Input: part model. Units: mm. Frame: model coordinates. A direction names the side the tool comes from. Round coordinates to 2 decimals unless told otherwise and drop trailing zeros. Loops run counter-clockwise (first coordinate to the right, second up) from the corner with the lowest first, then second, coordinate; pieces in that order, holes last. Notation, with made-up numbers: M -20.5,17 L 30.5,17 A23 cw 30.5,36 Z; hole C -37.5,-4 d2. An arc over 180 degrees is marked long. Use one line per item in the form item = value. Start each with the question number.
Q1. First-contact query: P1, Ø3, axis at x = -5, z = -6, coming from the +Y side; P2, Ø6, axis at y = 23.5, z = -13, coming from the -X side; P3, Ø4.5, axis at x = -4.5, z = -8.5, coming from the +Y side. Flat tips, straight axial feed; report the tip coordinate or a pass-through.
Q2. Section query A-A, the plane x = 0. Output: boundary loops of the cut face in (y, z), and give its area (3 significant figures).
Q3. Access query for faces 1 (the cylindrical face through (9.756, 13.804, -7.516)), 2 (the flat face through (0, 28, -11)). Directions: +Z, -Z, +X, -X, +Y, -Y. A direction counts if a zero-diameter tool reaches every point of the face in a straight line with its end or side. Return the directions, or none.
Q4. Section query D-D, the plane x = 4. Output: boundary loops of the cut face in (y, z), and give its area (3 significant figures).
Q5. Section query C-C, the plane y = 34. Output: boundary loops of the cut face in (x, z), and give its area (3 significant figures).
Q6. Section query B-B, the plane z = -7. Output: boundary loops of the cut face in (x, y).
Q7. Ray query, line 1 along Y through (x, z) = (6, -3.25); line 2 along X through (y, z) = (9.5, -7.5); line 3 along Y through (x, z) = (1, -5.5). Return the intervals inside material, ascending.
Autodesk Inventor part; units mm, degrees
ref_plane "YZ Plane" through (0, 0, 0) normal (1, 0, 0) x (0, 1, 0)
ref_plane "XZ Plane" through (0, 0, 0) normal (0, 1, 0) x (-1, 0, 0)
ref_plane "XY Plane" through (0, 0, 0) normal (0, 0, 1) x (1, 0, 0)
sketch "Sketch1" plane through (0, 0, 0) normal (0, 1, 0) x (-1, 0, 0)
  line L0 (0, 0) -> (-6.5, 0)
  line L1 (0, 0) -> (6.5, 0)
  line L2 (6.5, 0) -> (6.5, -15) construction
  line L3 (6.5, -15) -> (-7, -15)
  line L4 (-6.5, 0) -> (-9.5, 0) construction
  line L5 (6.5, 0) -> (9.5, 0) construction
  arc A0 (-6.5, 0) -> (-7, -15) centre (1.1167, -7.7622) ccw
  arc A1 (6.5, -15) -> (6.5, 0) centre (-1.375, -7.5) ccw
  dimension "d0" = 6.5
  dimension "d1" = 6.5
  dimension "d2" = 15
  dimension "d3" = 13.5
  dimension "d4" = 3
  dimension "d5" = 3
extrude "Extrusion1" add sketch "Sketch1" along normal blind 28
sketch "Sketch2" plane through (0, 28, 0) normal (0, 1, 0) x (1, 0, 0)
  line L0 (0, 0) -> (0, 7.5) construction
  circle A0 centre (0, 7.5) radius 3
  dimension "d8" = 7.5
  dimension "d9" = 6
extrude "Extrusion2" add sketch "Sketch2" along normal blind 1.6
sketch "Sketch3" plane through (0, 29.6, -7.5) normal (0, 1, 0) x (1, 0, 0)
  circle A0 centre (0, 0) radius 1
  point P0 (0, -7.5)
  dimension "d12" = 2
extrude "Extrusion3" add sketch "Sketch3" along normal blind 14
properties part number "FläktMotor"
Results found:
q1.P1 = 28
q1.P2 = -9.21
q1.P3 = 29.6
q2.outline = M 0,-15 L 28,-15 L 28,-10.5 L 29.6,-10.5 L 29.6,-8.5 L 43.6,-8.5 L 43.6,-6.5 L 29.6,-6.5 L 29.6,-4.5 L 28,-4.5 L 28,0 L 0,0 Z
q2.area = 458 mm²
q3.face_1 = +X, +Y, -Y
q3.face_2 = +Y
q4.outline = M 0,-15 L 28,-15 L 28,0 L 0,0 Z
q4.area = 420 mm²
q5.outline = C 0,-7.5 d2
q5.area = 3.14 mm²
q6.outline = M -9.49,0 L 9.73,0 L 9.73,28 L 2.96,28 L 2.96,29.6 L 0.87,29.6 L 0.87,43.6 L -0.87,43.6 L -0.87,29.6 L -2.96,29.6 L -2.96,28 L -9.49,28 Z
q7.line_1 = 0 to 28
q7.line_2 = -9.5 to 9.76
q7.line_3 = 0 to 29.6
